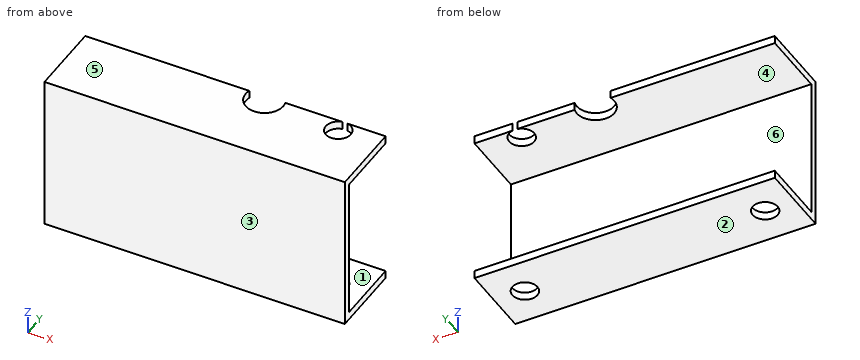
Autodesk Inventor part; units mm, degrees
ref_plane "YZ Plane" through (0, 0, 0) normal (1, 0, 0) x (0, 1, 0)
ref_plane "XZ Plane" through (0, 0, 0) normal (0, 1, 0) x (-1, 0, 0)
ref_plane "XY Plane" through (0, 0, 0) normal (0, 0, 1) x (1, 0, 0)
sketch "Sketch1" plane through (0, 0, 0) normal (1, 0, 0) x (0, 1, 0)
  line L0 (0, 0) -> (0, -40)
  line L1 (0, -40) -> (19, -40)
  line L2 (19, -40) -> (19, -38)
  line L3 (0, 0) -> (19, 0)
  line L4 (19, 0) -> (19, -2)
  line L5 (0, -20) -> (2, -20) construction
  line L6 (19, -2) -> (2, -2)
  line L7 (2, -2) -> (2, -38)
  line L8 (2, -38) -> (19, -38)
  dimension "d0" = 40
  dimension "d1" = 19
  dimension "d2" = 2
  dimension "d3" = 2
  dimension "d4" = 2
extrude "Extrusion1" add sketch "Sketch1" along normal blind 76.2
sketch "Sketch2" plane through (0, 2, -2) normal (0, 0, -1) x (-1, 0, 0)
  circle A0 centre (-65.9, 13.8784) radius 3.175
  point P0 (0, -2)
extrude "Extrusion2" cut sketch "Sketch2" against normal blind 25.4
sketch "Sketch3" plane through (0, 2, -2) normal (0, 0, -1) x (-1, 0, 0)
  circle A0 centre (-46.2, 15.7) radius 4.7625
  point P0 (0, -2)
extrude "Extrusion3" cut sketch "Sketch3" against normal blind 25.4
sketch "Sketch4" plane through (0, 0, -40) normal (0, 0, -1) x (-1, 0, 0)
  line L0 (-76.2, 9.5) -> (-68.58, 9.5) construction
  line L1 (-76.2, 9.5) -> (-68.58, 9.5) construction
  circle A0 centre (-68.58, 9.5) radius 3.175
  line L2 (0, 0) -> (0, 19)
  line L3 (0, 0) -> (-76.2, 0)
  line L4 (0, 9.5) -> (-7.62, 9.5) construction
  circle A1 centre (-7.62, 9.5) radius 3.175
  dimension "d11" = 7.62
  dimension "d12" = 6.35
  dimension "d15" = 7.62
  dimension "d16" = 6.35
extrude "Extrusion4" cut sketch "Sketch4" against normal blind 25.4
properties part number "3in C-Channel (TopPlate Supports)" material "Aluminum 6061"
Here's how the part is built. I have some questions about the finished solid (model axes, mm). Face numbers are marked on the shaded views. A direction names the side the tool comes from. Coordinates: 2 decimals unless noted, no trailing zeros. Loops run counter-clockwise (first coordinate to the right, second up) from the corner with the lowest first, then second, coordinate; pieces in that order, holes last. Notation, with made-up numbers: (-30, -37.5) - (-1, -37.5) arc R20 ccw to (-1, -26.5) - close; hole circle Ø11 at (-33.5, -1). An arc over 180 degrees is marked (long way). Return JSON: item names as keys, results as strings. Group by question number.
Item 1: Will these pins go through, and if not, where does the flat tip stop? P1, Ø5.5, axis at x = 7.62, y = 9.5, coming from the -Z side; P2, Ø11, axis at x = 46.5, z = -19, coming from the +Y side.
Item 2: We'd pull the mould along Z, two halves only. Please class the marked faces 3, 4, 5 and 6: +Z half, -Z half, draft (parallel to the pull), parting line (faces both ways), or undercut.
Item 3: If we section it at B-B on x = 7.62: Write out the boundary of the cut face in (y, z) (3 decimals), and give its area (3 significant figures).
Item 4: I need wall thicknesses on line 1 (Z direction, x = 20, y = 7); line 2 (Y direction, x = 68.58, z = -39) (3 decimals); line 3 (X direction, y = 17.7, z = -0.6). Which ranges of each line are inside material? Lowest first, please. Write a range as from..to.
Item 5: On a 3-axis mill with a long thin cutter (end or side, diameter ignored), from which of +Z, -Z, +X, -X, +Y, -Y can I reach the whole of each face in a straight line? I mean the marked faces 1 and 2. Say none if no direction works.
Item 6: If we section it at D-D on x = 46.2: Write out the boundary of the cut face in (y, z), and give its area (3 significant figures).
Item 7: If we section it at A-A on y = 3.75: Write out the boundary of the cut face in (x, z).
Item 8: If we section it at C-C on y = 9.5: Write out the boundary of the cut face in (x, z) (3 decimals).
Calculated:
{
 "1": {"P1": "stops at z = -2", "P2": "stops at y = 2"},
 "2": {"face 3": "draft", "face 4": "undercut", "face 5": "+Z half", "face 6": "undercut"},
 "3": {"outline": "(0, -40) - (6.325, -40) - (6.325, -38) - (2, -38) - (2, -2) - (19, -2) - (19, 0) - (0, 0) - close; (12.675, -40) - (19, -40) - (19, -38) - (12.675, -38) - close", "area": "135 mm^2"},
 "4": {"line 1": "z = -40..-38, -2..0", "line 2": "y = 0..6.325, 12.675..19", "line 3": "x = 0..41.44, 50.96..63.3, 68.5..76.2"},
 "5": {"face 1": "+X, -X, +Y", "face 2": "-Z, +X, -X, +Y, -Y"},
 "6": {"outline": "(0, -40) - (19, -40) - (19, -38) - (2, -38) - (2, -2) - (12.94, -2) - (12.94, 0) - (0, 0) - close", "area": "136 mm^2"},
 "7": {"outline": "(0, -40) - (76.2, -40) - (76.2, -38) - (0, -38) - close; (0, -2) - (76.2, -2) - (76.2, 0) - (0, 0) - close"},
 "8": {"outline": "(0, -40) - (4.445, -40) - (4.445, -38) - (0, -38) - close; (0, -2) - (76.2, -2) - (76.2, 0) - (0, 0) - close; (10.795, -40) - (65.405, -40) - (65.405, -38) - (10.795, -38) - close; (71.755, -40) - (76.2, -40) - (76.2, -38) - (71.755, -38) - close"}
}
